from build123d import *

# Parameters (mm, degrees)
SKETCH1_R               = 19.5
SKETCH1_R_2             = 17.5
BOSS_EXTRUDE1_DEPTH     = 37
BOSS_EXTRUDE2_START     = -2
SKETCH1_2_R             = 19.5
SKETCH1_2_R_2           = 17.5
BOSS_EXTRUDE2_DEPTH     = 2
CUT_EXTRUDE1_DEPTH      = 47.146505827
CUT_EXTRUDE1_DEPTH_BACK = 47.146505827
SKETCH2_R               = 5


with BuildPart() as part:
    # Sketch1 → Boss-Extrude1 (new body)
    with BuildSketch(Plane(origin=(0, 0, 0), x_dir=(1, 0, 0), z_dir=(0, 1, 0))):
        with Locations(Location((0, 0, 0), (0, 0, 270))):
            Circle(SKETCH1_R)
        with Locations(Location((0, 0, 0), (0, 0, 270))):
            Circle(SKETCH1_R_2, mode=Mode.SUBTRACT)
    extrude(amount=BOSS_EXTRUDE1_DEPTH)

    # Sketch1_2 → Boss-Extrude2 (add)
    # profile 1 of 2: a face of its own
    with BuildSketch(Plane(origin=(0, 0, 0), x_dir=(1, 0, 0), z_dir=(0, 1, 0)).offset(BOSS_EXTRUDE2_START)):
        with Locations(Location((0, 0, 0), (0, 0, 270))):
            Circle(SKETCH1_2_R)
        with Locations(Location((0, 0, 0), (0, 0, 270))):
            Circle(SKETCH1_2_R_2, mode=Mode.SUBTRACT)
    # profile 2 of 2: a face of its own
    with BuildSketch(Plane(origin=(0, 0, 0), x_dir=(1, 0, 0), z_dir=(0, 1, 0)).offset(BOSS_EXTRUDE2_START)):
        with Locations(Location((0, 0, 0), (0, 0, 270))):
            Circle(SKETCH1_2_R_2)
    extrude(amount=BOSS_EXTRUDE2_DEPTH)

    # Sketch2 → Cut-Extrude1 (cut, two sides: drawn at the far end of the back side and taken through both)
    with BuildSketch(Plane.XY.offset(-CUT_EXTRUDE1_DEPTH_BACK)):
        with Locations((0, 40)):
            Circle(SKETCH2_R)
    extrude(amount=CUT_EXTRUDE1_DEPTH + CUT_EXTRUDE1_DEPTH_BACK, mode=Mode.SUBTRACT)


solid = part.part
The listing builds one solid part. Answer for the finished solid, in the listing's coordinates (mm). A direction names the side the tool comes from. Give positions to 0.01 mm unless a question says otherwise; leave off trailing zeros. Write each loop counter-clockwise with the first axis right and the second up, starting at its lowest first coordinate (ties: lowest second). Pieces come first, ordered by that corner, then holes. Notation, with made-up numbers: (-5, -9) - (31, -9) arc R25 cw to (31, 24) - close; hole circle Ø10 at (-30.5, -34.75). An arc over 180 degrees is marked (long way). Use a Markdown table: item, result.
1. Find the intervals of material crossed by probe 1 along X at (y, z) = (22, 0); probe 2 along Y at (x, z) = (4.5, -6), in increasing order. Write a range as from..to.
Values follow:
| item | result |
|---|---|
| probe 1 | x = -19.5..-17.5, 17.5..19.5 |
| probe 2 | y = -2..0 |
2. Section A-A on z = 0 is taken. Write down the section's boundary in (x, y), plus the area to 3 significant figures.
Values follow:
| item | result |
|---|---|
| outline | (-19.5, -2) - (19.5, -2) - (19.5, 37) - (17.5, 37) - (17.5, 0) - (-17.5, 0) - (-17.5, 37) - (-19.5, 37) - close |
| area | 226 mm² |
3. Each of these flat-tipped pins is pushed along its axis until it touches: P1, Ø12, axis at y = 17.5, z = -10.5, coming from the +X side; P2, Ø6, axis at y = 13.5, z = -0.5, coming from the -X side; P3, Ø1.5, axis at x = 1.5, z = -9, coming from the +Y side. Where does it stop, or does it pass through?
Values follow:
| item | result |
|---|---|
| P1 | stops at x = 18.97 |
| P2 | stops at x = -19.5 |
| P3 | stops at y = 0 |
4. Section B-B on x = 0 is taken. Write down the section's boundary in (y, z).
Values follow:
| item | result |
|---|---|
| outline | (-2, -19.5) - (35, -19.5) - (35, -17.5) - (0, -17.5) - (0, 17.5) - (35, 17.5) - (35, 19.5) - (-2, 19.5) - close |
5. A tool of negligible diameter and unlimited length cuts with its end or side. For faces 4 (the flat face through (0, 0, 0)), 5 (the flat face through (18, 37, 0)), from which of +Z, -Z, +X, -X, +Y, -Y can it reach the whole face along a straight path? Write none if from no direction.
Values follow:
| item | result |
|---|---|
| face 4 | +Y |
| face 5 | +Z, -Z, +X, -X, +Y |
6. Section C-C on y = 3 is taken. Write down the section's boundary in (x, z).
Values follow:
| item | result |
|---|---|
| outline | circle Ø39 at (0, 0); hole circle Ø35 at (0, 0) |
7. For a pull along X with two mould halves and no side action, classify faces 1 (the cylindrical face through (19.334, 17.227, -2.539)), 2 (the cylindrical face through (0, 35, 18)), 3 (the flat face through (0, -2, 0)) as released by +X, released by -X, zero draft, split by the parting line, or undercut.
Values follow:
| item | result |
|---|---|
| face 1 | split by the parting line |
| face 2 | undercut |
| face 3 | zero draft |
